```python
from build123d import *

# Parameters (mm, degrees)
F0_R     = 28.5834260478
F1_DEPTH = 25.4


with BuildPart() as f1:
    # F0 (on Front) → F1 (new body)
    with BuildSketch(Plane.XZ):
        with BuildLine():
            Line((0, -111.1967209602), (0, 0))
            Line((0, 0), (0, 10.4824639664))
            ThreePointArc((0, 10.4824639664), (-28.5834260478, 39.0658900142), (0, 67.6493160619))
            Line((0, 67.6493160619), (0, 189.3285009885))
            ThreePointArc((0, 189.3285009885), (-85.6264774345, 162.5444655606), (-140.7274290539, 91.7407698783))
            Line((-140.7274290539, 91.7407698783), (-148.9322934456, 19.1153455136))
            ThreePointArc((-148.9322934456, 19.1153455136), (-98.9470346949, -74.0196377156), (0, -111.1967209602))
        make_face()
        with BuildLine():
            Line((0, 10.4824639664), (0, 0))
            Line((0, 0), (0, -111.1967209602))
            ThreePointArc((0, -111.1967209602), (99.7081962508, -73.3490905589), (149.1880764193, 21.1279383162))
            Line((149.1880764193, 21.1279383162), (141.38502058, 89.9493668256))
            ThreePointArc((141.38502058, 89.9493668256), (86.4088195027, 161.9982623535), (0, 189.3285009885))
            Line((0, 189.3285009885), (0, 67.6493160619))
            ThreePointArc((0, 67.6493160619), (20.2115343879, 59.2774244021), (28.5834260478, 39.0658900142))
            ThreePointArc((28.5834260478, 39.0658900142), (20.2115343879, 18.8543556262), (0, 10.4824639664))
        make_face()
        with BuildLine():
            ThreePointArc((149.1880764193, 21.1279383162), (99.7081962508, -73.3490905589), (0, -111.1967209602))
            Line((0, -111.1967209602), (0, -252.5826123669))
            Line((0, -252.5826123669), (118.9536322579, -252.5826123669))
            Line((118.9536322579, -252.5826123669), (149.1880764193, 21.1279383162))
        make_face()
        with BuildLine():
            Line((0, -252.5826123669), (0, -111.1967209602))
            ThreePointArc((0, -111.1967209602), (-98.9470346949, -74.0196377156), (-148.9322934456, 19.1153455136))
            Line((-148.9322934456, 19.1153455136), (-105.8942795707, -370.8081200368))
            ThreePointArc((-105.8942795707, -370.8081200368), (-79.3581582284, -288.0390857098), (0, -252.5826123669))
        make_face()
        with BuildLine():
            Line((118.9536322579, -252.5826123669), (0, -252.5826123669))
            ThreePointArc((0, -252.5826123669), (75.3332961831, -283.7866853442), (106.5373691604, -359.1199815273))
            Line((106.5373691604, -359.1199815273), (107.1853678233, -359.1199815273))
            Line((107.1853678233, -359.1199815273), (118.9536322579, -252.5826123669))
        make_face()
        with BuildLine():
            Line((0, -330.5365554796), (0, -252.5826123669))
            ThreePointArc((0, -252.5826123669), (-79.3581582284, -288.0390857098), (-105.8942795707, -370.8081200368))
            ThreePointArc((-105.8942795707, -370.8081200368), (-71.0808958175, -438.4781397557), (0, -465.6573506877))
            ThreePointArc((0, -465.6573506877), (75.3332961831, -434.4532777104), (106.5373691604, -359.1199815273))
            Line((106.5373691604, -359.1199815273), (28.5834260478, -359.1199815273))
            ThreePointArc((28.5834260478, -359.1199815273), (-20.2115343879, -379.3315159153), (0, -330.5365554796))
        make_face()
        with BuildLine():
            ThreePointArc((-140.7274290539, 91.7407698783), (-149.3127649454, 55.9345141776), (-148.9322934456, 19.1153455136))
            Line((-148.9322934456, 19.1153455136), (-140.7274290539, 91.7407698783))
        make_face()
        with BuildLine():
            Line((141.38502058, 89.9493668256), (149.1880764193, 21.1279383162))
            ThreePointArc((149.1880764193, 21.1279383162), (149.993736779, 30.0808366528), (150.2626109743, 39.0658900142))
            ThreePointArc((150.2626109743, 39.0658900142), (148.0265763332, 64.891941898), (141.38502058, 89.9493668256))
        make_face()
        with BuildLine():
            ThreePointArc((-140.7274290539, 91.7407698783), (-85.6264774345, 162.5444655606), (0, 189.3285009885))
            Line((0, 189.3285009885), (0, 284.7426560834))
            ThreePointArc((0, 284.7426560834), (-76.6118719963, 317.2473831402), (-106.4749269686, 394.9270726321))
            Line((-106.4749269686, 394.9270726321), (-140.7274290539, 91.7407698783))
        make_face()
        with Locations((-46.7894114554, 249.1482943296)):
            Circle(F0_R, mode=Mode.SUBTRACT)
        with BuildLine():
            Line((0, 284.7426560834), (0, 189.3285009885))
            ThreePointArc((0, 189.3285009885), (86.4088195027, 161.9982623535), (141.38502058, 89.9493668256))
            Line((141.38502058, 89.9493668256), (105.8807391162, 403.0901950914))
            ThreePointArc((105.8807391162, 403.0901950914), (106.3730849835, 397.1942300687), (106.5373691604, 391.2800252438))
            ThreePointArc((106.5373691604, 391.2800252438), (75.3332961831, 315.9467290607), (0, 284.7426560834))
        make_face()
        with BuildLine():
            Line((107.1853678233, -359.1199815273), (106.5373691604, -359.1199815273))
            ThreePointArc((106.5373691604, -359.1199815273), (75.3332961831, -434.4532777104), (0, -465.6573506877))
            Line((0, -465.6573506877), (358.4000170231, -465.6573506877))
            ThreePointArc((358.4000170231, -465.6573506877), (283.06672084, -434.4532777104), (251.8626478627, -359.1199815273))
            Line((251.8626478627, -359.1199815273), (107.1853678233, -359.1199815273))
        make_face()
        with BuildLine():
            Line((358.4000170231, -252.5826123669), (118.9536322579, -252.5826123669))
            Line((118.9536322579, -252.5826123669), (107.1853678233, -359.1199815273))
            Line((107.1853678233, -359.1199815273), (251.8626478627, -359.1199815273))
            ThreePointArc((251.8626478627, -359.1199815273), (283.06672084, -283.7866853442), (358.4000170231, -252.5826123669))
        make_face()
        with BuildLine():
            ThreePointArc((-106.4749269686, 394.9270726321), (-76.6118719963, 317.2473831402), (0, 284.7426560834))
            ThreePointArc((0, 284.7426560834), (75.3332961831, 315.9467290607), (106.5373691604, 391.2800252438))
            ThreePointArc((106.5373691604, 391.2800252438), (106.3730849835, 397.1942300687), (105.8807391162, 403.0901950914))
            ThreePointArc((105.8807391162, 403.0901950914), (4.2430021395, 497.7328690783), (-104.6048877063, 411.4797404785))
            Line((-104.6048877063, 411.4797404785), (-106.4749269686, 394.9270726321))
        make_face()
        with BuildLine():
            ThreePointArc((28.5834260478, 391.2800252438), (20.2115343879, 371.0684908558), (0, 362.696599196))
            ThreePointArc((0, 362.696599196), (-20.2115343879, 411.4915596317), (28.5834260478, 391.2800252438))
        make_face(mode=Mode.SUBTRACT)
        with BuildLine():
            ThreePointArc((464.9373861835, -359.1199815273), (433.7333132062, -283.7866853442), (358.4000170231, -252.5826123669))
            ThreePointArc((358.4000170231, -252.5826123669), (283.06672084, -283.7866853442), (251.8626478627, -359.1199815273))
            ThreePointArc((251.8626478627, -359.1199815273), (283.06672084, -434.4532777104), (358.4000170231, -465.6573506877))
            ThreePointArc((358.4000170231, -465.6573506877), (433.7333132062, -434.4532777104), (464.9373861835, -359.1199815273))
        make_face()
        with BuildLine():
            ThreePointArc((386.9834430709, -359.1199815273), (358.4000170231, -387.7034075751), (329.8165909753, -359.1199815273))
            ThreePointArc((329.8165909753, -359.1199815273), (358.4000170231, -330.5365554796), (386.9834430709, -359.1199815273))
        make_face(mode=Mode.SUBTRACT)
        with BuildLine():
            ThreePointArc((-104.6048877063, 411.4797404785), (-105.8639208796, 403.2400120168), (-106.4749269686, 394.9270726321))
            Line((-106.4749269686, 394.9270726321), (-104.6048877063, 411.4797404785))
        make_face()
        with BuildLine():
            ThreePointArc((106.5373691604, -359.1199815273), (75.3332961831, -283.7866853442), (0, -252.5826123669))
            Line((0, -252.5826123669), (0, -330.5365554796))
            ThreePointArc((0, -330.5365554796), (20.2115343879, -338.9084471394), (28.5834260478, -359.1199815273))
            Line((28.5834260478, -359.1199815273), (106.5373691604, -359.1199815273))
        make_face()
    extrude(amount=F1_DEPTH)


solid = f1.part
```
Can you work these out from the model? Positions are in its coordinate system, mm. Coordinates: 2 decimals unless noted, no trailing zeros. Loops run counter-clockwise (first coordinate to the right, second up) from the corner with the lowest first, then second, coordinate; pieces in that order, holes last.
1) I need wall thicknesses on probe 1 along X at (y, z) = (-8.25, 37.5); probe 2 along Z at (x, y) = (244, -13.5); probe 3 along X at (y, z) = (-13.5, 420). Which ranges of each line are inside material? Lowest first, please.
2) Imagine slicing it at C-C on z = 142.5. List the corners of the cut face in (x, y) for me, plus the area to 3 significant figures.
3) Thinking about a two-plate mould opening in X: for faces 1 (the flat face through (133.86, -12.52, -117.64)), 2 (the cylindrical face through (-1.257, -12.522, 419.836)), 3 (the cylindrical face through (-71.889, -12.522, -437.747)), 4 (the cylindrical face through (-10.948, -12.522, -332.716)), which applies, pulls with the +X half, pulls with the -X half, needs draft (parallel to the pull), parting line crosses it, or undercut?
4) For pin 1 (4 mm diameter, centred on x = 269, y = -3.5, fed in from +Z); pin 2 (12 mm diameter, centred on x = -15, y = -4.5, fed in from -Z); pin 3 (6 mm diameter, centred on x = 382, y = -4, fed in from -Z); pin 4 (4 mm diameter, centred on x = 10, z = -41.5, fed in from +Y), each with a flat end and sliding along its axis, tell me the tip position at first contact or that it passes through.
5) Imagine slicing it at B-B on y = -21. List the corners of the cut face in (x, z) for me, plus the area to 3 significant figures.
6) Imagine slicing it at A-A on x = 341. List the corners of the cut face in (y, z) for me, plus the area to 3 significant figures.
7) Imagine slicing it at D-D on x = 64. List the corners of the cut face in (y, z) for me, plus the area to 3 significant figures.
Completed:
1. probe 1: x = -150.25 to -28.54, 28.54 to 150.25
1. probe 2: z = -465.66 to -252.58
1. probe 3: x = -102.59 to 102.59
2. outline: (-134.99, -25.4) - (135.43, -25.4) - (135.43, 0) - (-134.99, 0) - close
2. area: 6,870 mm2
3. face 1: pulls with the +X half
3. face 2: undercut
3. face 3: pulls with the -X half
3. face 4: undercut
4. pin 1: stops at z = -252.58
4. pin 2: stops at z = -465.28
4. pin 3: stops at z = -463.65
4. pin 4: stops at y = 0
5. outline: (-148.93, 19.12) - (-105.89, -370.81) arc R106.54 ccw to (0, -465.66) - (358.4, -465.66) arc R106.54 ccw to (358.4, -252.58) - (118.95, -252.58) - (149.19, 21.13) arc R150.26 ccw to (141.39, 89.95) - (105.88, 403.09) arc R106.54 ccw to (-106.47, 394.93) - (-140.73, 91.74) arc R150.26 ccw to start; hole circle Ø57.17 at (-46.79, 249.15); hole circle Ø57.17 at (0, -359.12); hole circle Ø57.17 at (0, 39.07); hole circle Ø57.17 at (0, 391.28); hole circle Ø57.17 at (358.4, -359.12)
5. area: 289,000 mm2
6. outline: (-25.4, -465.66) - (0, -465.66) - (0, -381.8) - (-25.4, -381.8) - close; (-25.4, -336.44) - (0, -336.44) - (0, -252.58) - (-25.4, -252.58) - close
6. area: 4,260 mm2
7. outline: (-25.4, -465.66) - (0, -465.66) - (0, 476.45) - (-25.4, 476.45) - close
7. area: 23,900 mm2
